Print and shaded views of the part. All mm, measured from the part's lowest x, y and z. Round coordinates to 2 decimals unless told otherwise and drop trailing zeros. Order: outer loops, then holes, each group sorted by start corner. A loop starts at its lowest first (then second) coordinate and runs counter-clockwise, first axis right, second up. Notation, with made-up numbers: (89, 16.5) - (125, 16.5) arc R23 ccw to (125, 26.5) - close; hole circle Ø8 at (42.25, -7.5). An arc over 180 degrees is marked (long way). Return JSON: item names as keys, results as strings. Group by question number.
Item 1: Probe probe 1 along Y at (x, z) = (30, 0.7); probe 2 along Y at (x, z) = (17.5, 1.1); probe 3 along X at (y, z) = (29, 1.3). List the from-to ranges inside material, lowest first.
Item 2: Drop flat-ended pins along their axis: pin 1 (6 mm diameter, centred on x = 8.5, y = 10.5, fed in from -Z); pin 2 (2.5 mm diameter, centred on x = 30, y = 30, fed in from +Z). Give the stop position or say it passes through.
Item 3: Saw through at B-B on x = 6. List the corners of the cut face in (y, z), and give its area (3 significant figures).
Item 4: Saw through at A-A on z = 0.5. List the corners of the cut face in (x, y).
Item 5: Saw through at D-D on x = 17. List the corners of the cut face in (y, z).
Item 6: Saw through at C-C on y = 17.5. List the corners of the cut face in (x, z).
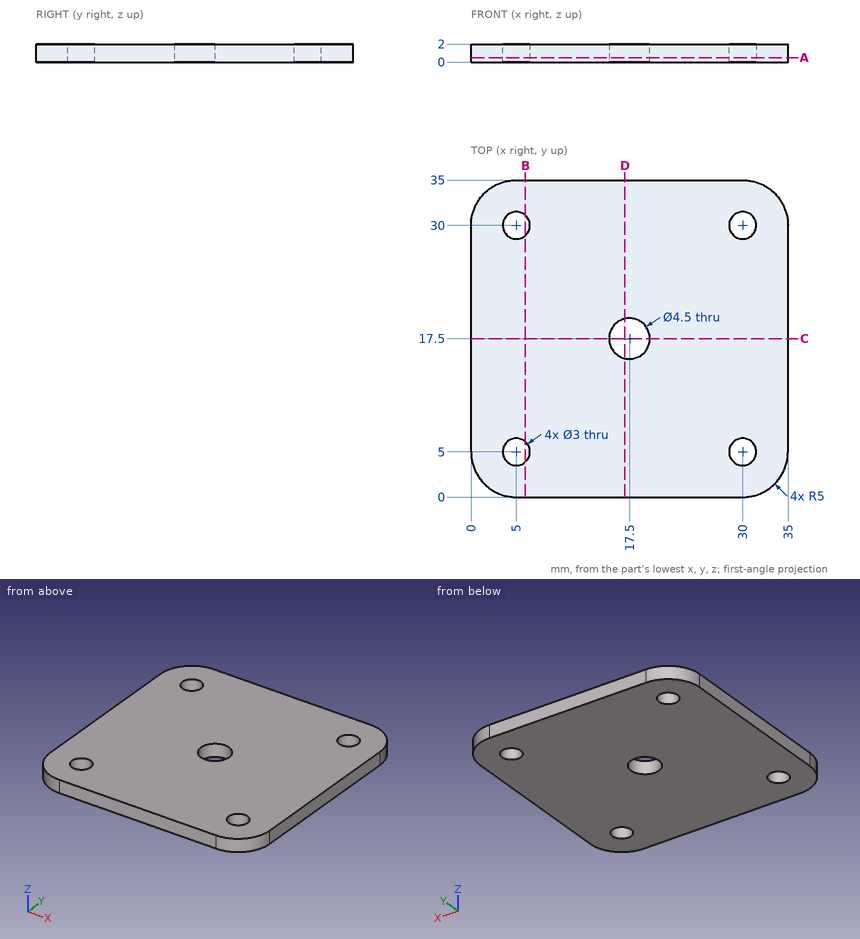
Filled in:
{
 "1": {"probe 1": "y = 0 to 3.5, 6.5 to 28.5, 31.5 to 35", "probe 2": "y = 0 to 15.25, 19.75 to 35", "probe 3": "x = 0 to 3.88, 6.12 to 28.88, 31.12 to 35"},
 "2": {"pin 1": "stops at z = 0", "pin 2": "passes through"},
 "3": {"outline": "(0, 0) - (3.88, 0) - (3.88, 2) - (0, 2) - close; (6.12, 0) - (28.88, 0) - (28.88, 2) - (6.12, 2) - close; (31.12, 0) - (35, 0) - (35, 2) - (31.12, 2) - close", "area": "61.1 mm^2"},
 "4": {"outline": "(0, 5) arc R5 ccw to (5, 0) - (30, 0) arc R5 ccw to (35, 5) - (35, 30) arc R5 ccw to (30, 35) - (5, 35) arc R5 ccw to (0, 30) - close; hole circle Ø3 at (5, 5); hole circle Ø3 at (5, 30); hole circle Ø4.5 at (17.5, 17.5); hole circle Ø3 at (30, 5); hole circle Ø3 at (30, 30)"},
 "5": {"outline": "(0, 0) - (15.31, 0) - (15.31, 2) - (0, 2) - close; (19.69, 0) - (35, 0) - (35, 2) - (19.69, 2) - close"},
 "6": {"outline": "(0, 0) - (15.25, 0) - (15.25, 2) - (0, 2) - close; (19.75, 0) - (35, 0) - (35, 2) - (19.75, 2) - close"}
}
